Source: CAD feature listing. Evaluate the final solid. Frame: model axes, mm. Coordinates: 2 decimals unless noted, no trailing zeros. Order: outer loops, then holes, each group sorted by start corner. A loop starts at its lowest first (then second) coordinate and runs counter-clockwise, first axis right, second up.
Item 1: Ray query, line 1 (Z direction, x = 2.35, y = 8); line 2 (Y direction, x = 2, z = -115) (3 decimals); line 3 (Z direction, x = 0.35, y = 33.5). Return the intervals inside material, ascending.
Item 2: Section B-B on y = 31.5. Return the cut outline in (x, z), then the cut area to 3 significant figures.
Item 3: Section A-A on z = -5. Return the cut outline in (x, y) (3 decimals).
Item 4: Section C-C on z = -41.5. Return the cut outline in (x, y), then the cut area to 3 significant figures.
Item 5: Contact query for flat-ended pins moving along their axis: P1, Ø4, axis at y = 42.695, z = -5, coming from the -X side; P2, Ø1.5, axis at x = 1.5, z = -106, coming from the -Y side; P3, Ø0.9, axis at x = 1, z = -5.5, coming from the -Y side. Output: stop coordinate, or through.
from build123d import *

# Parameters (mm, degrees)
SKETCH2_W                      = 3
SKETCH2_H                      = 10.78
BOSS_EXTRUDE2_DEPTH            = 3
HOLE_FOR_M3_300_SC_NUTS_SP_1_D = 4.22
SKETCH10_R                     = 8
CUT_EXTRUDE1_DEPTH             = 10


with BuildPart() as part:
    # Sketch2 → Boss-Extrude2 (new body)
    with BuildSketch(Plane(origin=(0, 0, 0), x_dir=(0, 0, -1), z_dir=(1, 0, 0))):
        Polygon((0, 0), (2.89, 0), (2.89, 5), (2.5, 5), (2.5, 7), (2.89, 7), (2.89, 10), (7.11, 10), (7.11, 7), (7.5, 7), (7.5, 5), (7.11, 5), (7.11, 0), (17.11, 0), (17.11, -3), (47.89, -3), (47.89, 0), (57.89, 0), (57.89, 5), (57.5, 5), (57.5, 7), (57.89, 7), (57.89, 10), (62.11, 10), (62.11, 7), (62.5, 7), (62.5, 5), (62.11, 5), (62.11, 0), (72.11, 0), (72.11, -3), (102.89, -3), (102.89, 0), (112.89, 0), (112.89, 5), (112.5, 5), (112.5, 7), (112.89, 7), (112.89, 10), (117.11, 10), (117.11, 7), (117.5, 7), (117.5, 5), (117.11, 5), (117.11, 0), (120, 0), (120, 50), (0, 50), align=None)
        with Locations((115, 30)):
            Rectangle(SKETCH2_W, SKETCH2_H, mode=Mode.SUBTRACT)
        with Locations((5, 30)):
            Rectangle(SKETCH2_W, SKETCH2_H, mode=Mode.SUBTRACT)
    extrude(amount=BOSS_EXTRUDE2_DEPTH)

    # Hole for M3 300® SC Nuts (SP)1 (through all)
    with Locations(Plane(origin=(3, 0, 0), x_dir=(0, 0, -1), z_dir=(1, 0, 0))):
        with Locations((5, 42.695), (5, 17.305), (115, 42.695), (115, 17.305)):
            Hole(HOLE_FOR_M3_300_SC_NUTS_SP_1_D / 2)

    # Sketch10 → Cut-Extrude1 (cut)
    with BuildSketch(Plane(origin=(3, 0, 0), x_dir=(0, 0, -1), z_dir=(1, 0, 0))):
        with Locations((73, 25)):
            Circle(SKETCH10_R)
        with Locations((47, 25)):
            Circle(SKETCH10_R)
    extrude(amount=-CUT_EXTRUDE1_DEPTH, mode=Mode.SUBTRACT)


solid = part.part
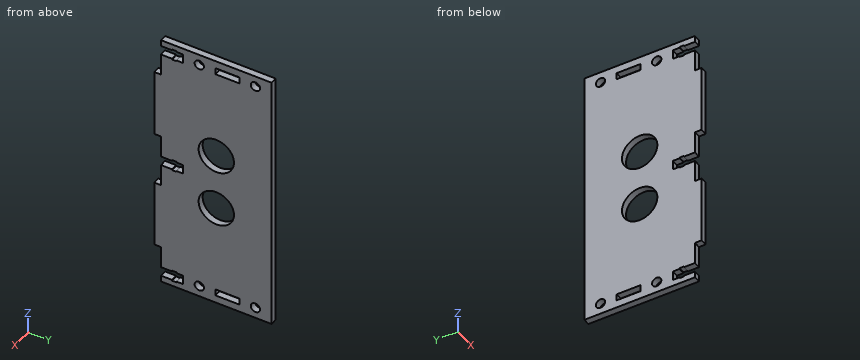
Answer list:
1. line 1: z = -120 to -117.11, -112.89 to -62.11, -57.89 to -7.11, -2.89 to 0
1. line 2: y = 10 to 15.195, 19.415 to 24.61, 35.39 to 40.585, 44.805 to 50
1. line 3: z = -120 to -116.5, -113.5 to -6.5, -3.5 to 0
2. outline: (0, -120) - (3, -120) - (3, -116.5) - (0, -116.5) - close; (0, -113.5) - (3, -113.5) - (3, -77.66) - (0, -77.66) - close; (0, -68.34) - (3, -68.34) - (3, -51.66) - (0, -51.66) - close; (0, -42.34) - (3, -42.34) - (3, -6.5) - (0, -6.5) - close; (0, -3.5) - (3, -3.5) - (3, 0) - (0, 0) - close
2. area: 286 mm2
3. outline: (0, 10) - (3, 10) - (3, 15.195) - (0, 15.195) - close; (0, 19.415) - (3, 19.415) - (3, 24.61) - (0, 24.61) - close; (0, 35.39) - (3, 35.39) - (3, 40.585) - (0, 40.585) - close; (0, 44.805) - (3, 44.805) - (3, 50) - (0, 50) - close
4. outline: (0, -3) - (3, -3) - (3, 19.19) - (0, 19.19) - close; (0, 30.81) - (3, 30.81) - (3, 50) - (0, 50) - close
4. area: 124 mm2
5. P1: passes through
5. P2: stops at y = 0
5. P3: stops at y = 10
